```python
from build123d import *

# Parameters (mm, degrees)
F1_DEPTH = 6.35


with BuildPart() as f1:
    # F0 (on Front) → F1 (new body)
    with BuildSketch(Plane.XZ):
        with BuildLine():
            Line((-5.524762, 0), (-0.508, 0))
            ThreePointArc((-0.508, 0), (-0.14879, 0.14879), (0, 0.508))
            Line((0, 0.508), (0, 15.367))
            ThreePointArc((0, 15.367), (-0.14879, 15.72621), (-0.508, 15.875))
            Line((-0.508, 15.875), (-4.445, 15.875))
            ThreePointArc((-4.445, 15.875), (-6.318154, 14.316871), (-5.127144, 12.191319))
            ThreePointArc((-5.127144, 12.191319), (-4.677356, 11.664932), (-4.873952, 11.001048))
            Line((-4.873952, 11.001048), (-5.964836, 9.910164))
            ThreePointArc((-5.964836, 9.910164), (-6.023912, 9.643686), (-5.807368, 9.477526))
            Line((-5.807368, 9.477526), (-4.828483, 9.391884))
            ThreePointArc((-4.828483, 9.391884), (-3.240143, 8.070876), (-3.921246, 6.120495))
            Line((-3.921246, 6.120495), (-4.264111, 5.871389))
            ThreePointArc((-4.264111, 5.871389), (-4.45948, 5.341818), (-4.044985, 4.958663))
            Line((-4.044985, 4.958663), (-2.379395, 4.694859))
            ThreePointArc((-2.379395, 4.694859), (-1.597478, 3.960691), (-1.992111, 2.963365))
            Line((-1.992111, 2.963365), (-5.667589, 0.464039))
            ThreePointArc((-5.667589, 0.464039), (-5.767524, 0.17928), (-5.524762, 0))
        make_face()
    extrude(amount=F1_DEPTH)


solid = f1.part
```
Can you work these out from the model? Positions are in its coordinate system, mm. A direction names the side the tool comes from. Give positions to 0.01 mm unless a question says otherwise; leave off trailing zeros. Write each loop counter-clockwise with the first axis right and the second up, starting at its lowest first coordinate (ties: lowest second). Pieces come first, ordered by that corner, then holes. Notation, with made-up numbers: (6.5, 77.5) -> (29.5, 77.5) arc R29 ccw to (29.5, 105.5) -> close; hole circle Ø9 at (65, 34.25). An arc over 180 degrees is marked (long way). Write item = value, one per line.
(1) Suppose I cut it at D-D on z = 7.25. Write out the boundary of the cut face in (x, y).
Worked out:
outline = (-3.21, -6.35) -> (0, -6.35) -> (0, 0) -> (-3.21, 0) -> close
(2) I'm going to push a flat-ended pin straight in: P1, Ø2, axis at y = -4.5, z = 2, coming from the -X side. Where does the tip first touch, or does it pass through?
Worked out:
P1 = -4.88
(3) Suppose I cut it at A-A on y = -3.25. Write out the boundary of the cut face in (x, z) (1 decimal).
Worked out:
outline = (-6, 9.9) arc R0.3 ccw to (-5.8, 9.5) -> (-4.8, 9.4) arc R1.8 cw to (-3.9, 6.1) -> (-4.3, 5.9) arc R0.5 ccw to (-4, 5) -> (-2.4, 4.7) arc R1 cw to (-2, 3) -> (-5.7, 0.5) arc R0.3 ccw to (-5.5, 0) -> (-0.5, 0) arc R0.5 ccw to (0, 0.5) -> (0, 15.4) arc R0.5 ccw to (-0.5, 15.9) -> (-4.4, 15.9) arc R1.9 ccw to (-5.1, 12.2) arc R0.7 cw to (-4.9, 11) -> close
(4) Thinking about a two-plate mould opening in Z: for faces 1 (the face through (-3.25, -3.13, 8.1)), 2 (the face through (-4.68, -3.13, 11.67)), 3 (the face through (-2, -3, 15.875)), 4 (the face through (-3, -6.35, 10)), which applies, released by +Z, released by -Z, zero draft, split by the parting line, or undercut?
Worked out:
face_1 = undercut
face_2 = undercut
face_3 = released by +Z
face_4 = zero draft
(5) For faces 5 (the face through (-3.22, -3.13, 4.83)), 6 (the face through (-3, 0, 10)), which set-ups out of +Z, -Z, +X, -X, +Y, -Y let a thin tool reach every point of the face, with its end or its side?
Worked out:
face_5 = -X, +Y, -Y
face_6 = +Z, -Z, +X, -X, +Y
(6) Suppose I cut it at C-C on x = -1.75. Write out the boundary of the cut face in (y, z) (3 decimals).
Worked out:
outline = (-6.35, 0) -> (0, 0) -> (0, 3.201) -> (-6.35, 3.201) -> close; (-6.35, 4.304) -> (0, 4.304) -> (0, 15.875) -> (-6.35, 15.875) -> close
(7) I need wall thicknesses on probe 1 along Z at (x, y) = (-3.5, -0.5) (3 decimals); probe 2 along Z at (x, y) = (-4, -2.25) (3 decimals); probe 3 along Z at (x, y) = (-2.5, -4.75) (3 decimals). Which ranges of each line are inside material? Lowest first, please. Write a range as from..to.
Worked out:
probe_1 = 0..1.938, 4.872..6.55, 8.623..15.875
probe_2 = 0..1.598, 4.952..6.063, 9.107..15.875
probe_3 = 0..2.618, 4.714..15.875
(8) Suppose I cut it at B-B on x = -3.5. Write out the boundary of the cut face in (y, z) (3 decimals), then the cut area to 3 significant figures.
Worked out:
outline = (-6.35, 0) -> (0, 0) -> (0, 1.938) -> (-6.35, 1.938) -> close; (-6.35, 4.872) -> (0, 4.872) -> (0, 6.55) -> (-6.35, 6.55) -> close; (-6.35, 8.623) -> (0, 8.623) -> (0, 15.875) -> (-6.35, 15.875) -> close
area = 69.0 mm^2
